Could you check a few things on this model? Use its own coordinates, in mm. A direction names the side the tool comes from. Round coordinates to 2 decimals unless told otherwise and drop trailing zeros. Write each loop counter-clockwise with the first axis right and the second up, starting at its lowest first coordinate (ties: lowest second). Pieces come first, ordered by that corner, then holes. Notation, with made-up numbers: (85, -31.75) -> (107, -31.75) arc R17 ccw to (107, -21.75) -> close; hole circle Ø6 at (32, 32.25). An arc over 180 degrees is marked (long way). Return JSON: item names as keys, results as strings.
from build123d import *

# Parameters (mm, degrees)
PAD_DEPTH = 8
FILLET_R  = 1


with BuildPart() as part:
    # Sketch → Pad (new body)
    with BuildSketch(Plane.XY):
        Polygon((0, 0), (0, 47), (10, 47), (10, 52), (-25, 52), (-25, -5), (4, -5), (4, 0), align=None)
    extrude(amount=PAD_DEPTH)

    # Fillet
    fillet_edges = [part.edges().sort_by_distance(p)[0] for p in [
        (-25, 52, 4),
        (-25, -5, 4),
        (10, 52, 4),
    ]]
    fillet(fillet_edges, radius=FILLET_R)


solid = part.part
1) Will these pins go through, and if not, where does the flat tip stop? pin 1 Ø2.5 at (y, z) = (-2, 2.5) entering from +X; pin 2 Ø4 at (y, z) = (32, 2.5) entering from +X.
Return value:
{"pin 1": "x = 4", "pin 2": "x = 0"}
2) Thinking about a two-plate mould opening in Y: for faces 1 (the face through (4, -3, 4)), 2 (the face through (-7, 52, 4)), 3 (the face through (2, 0, 4)), 4 (the face through (-10, -5, 4)), which applies, pulls with the +Y half, pulls with the -Y half, needs draft (parallel to the pull), parting line crosses it, or undercut?
Return value:
{"face 1": "needs draft", "face 2": "pulls with the +Y half", "face 3": "undercut", "face 4": "pulls with the -Y half"}
3) I want a section at B-B, the plane y = 34.5. Please give me the cut outline in (x, z), and give its area (3 significant figures).
Return value:
{"outline": "(-25, 0) -> (0, 0) -> (0, 8) -> (-25, 8) -> close", "area": "200 mm²"}
4) If I drill on probe 1 along Y at (x, z) = (2, 4); probe 2 along X at (y, z) = (6.5, 5.5); probe 3 along X at (y, z) = (-1, 7), over which ranges is the centre line in solid material (lowest first)? Write a range as [from, to].
Return value:
{"probe 1": "[-5, 0], [47, 52]", "probe 2": "[-25, 0]", "probe 3": "[-25, 4]"}
5) I want a section at A-A, the plane z = 4.25. Please give me the cut outline in (x, y).
Return value:
{"outline": "(-25, -4) arc R1 ccw to (-24, -5) -> (4, -5) -> (4, 0) -> (0, 0) -> (0, 47) -> (10, 47) -> (10, 51) arc R1 ccw to (9, 52) -> (-24, 52) arc R1 ccw to (-25, 51) -> close"}
6) For faces 5 (the face through (5, 47, 4)), 6 (the face through (10, 49, 4)), which set-ups out of +Z, -Z, +X, -X, +Y, -Y let a thin tool reach every point of the face, with its end or its side?
Return value:
{"face 5": "+Z, -Z, +X", "face 6": "+Z, -Z, +X, +Y, -Y"}
